```python
from build123d import *

# Parameters (mm, degrees)
EXTRUDE_THIN1_DEPTH = 100
CUT_EXTRUDE2_DEPTH  = 33.5
FILLET1_R           = 3
SKETCH6_W           = 108.670856817
SKETCH6_H           = 17.879774232
CUT_EXTRUDE3_DEPTH  = 166
BOSS_EXTRUDE1_DEPTH = 10.5
CUT_EXTRUDE4_DEPTH  = 27
CUT_EXTRUDE7_DEPTH  = 5
FILLET5_R           = 12


with BuildPart() as part:
    # Sketch1 → Extrude-Thin1 (new body)
    with BuildSketch(Plane(origin=(0, 0, 0), x_dir=(0, 0, -1), z_dir=(1, 0, 0))):
        with BuildLine():
            Line((45, -32), (45, -18))
            ThreePointArc((45, -18), (32.040658091, -6.957616726), (16.501342128, 0))
            ThreePointArc((16.501342128, 0), (0, 1.972757604), (-16.501342128, 0))
            ThreePointArc((-16.501342128, 0), (-32.040658091, -6.957616726), (-45, -18))
            Line((-45, -18), (-45, -32))
            Line((-45, -32), (-48, -32))
            Line((-48, -32), (-48, -16.88185814))
            ThreePointArc((-48, -16.88185814), (-34.099982932, -4.712774746), (-17.26768466, 2.901081048))
            ThreePointArc((-17.26768466, 2.901081048), (0, 4.972757604), (17.26768466, 2.901081048))
            ThreePointArc((17.26768466, 2.901081048), (34.099982932, -4.712774746), (48, -16.88185814))
            Line((48, -16.88185814), (48, -32))
            Line((48, -32), (45, -32))
        make_face()
    extrude(amount=EXTRUDE_THIN1_DEPTH)

    # Sketch5 → Cut-Extrude2 (cut, symmetric)
    with BuildSketch(Plane(origin=(0, 0, 0), x_dir=(1, 0, 0), z_dir=(0, 1, 0))):
        with BuildLine():
            Line((74.78082212, 3), (74.78082212, -3))
            add(Edge.make_bspline(
                [(74.78082212, -3), (97.634090292, -10.562952057), (100, -44)],
                knots=[0, 0, 0, 1, 1, 1], degree=2))
            Line((100, -44), (100, 44))
            add(Edge.make_bspline(
                [(74.78082212, 3), (97.634090292, 10.562952057), (100, 44)],
                knots=[0, 0, 0, 1, 1, 1], degree=2))
        make_face()
    extrude(amount=CUT_EXTRUDE2_DEPTH, both=True, mode=Mode.SUBTRACT)

    # Fillet1
    fillet1_edges = [part.edges().sort_by_distance(p)[0] for p in [
        (50, -16.88185814, -48),
        (50, -16.88185814, 48),
        (74.78082212, 3.409765032, 3),
        (74.78082212, 3.409765032, -3),
        (46.328171757, 2.901081048, -17.26768466),
        (46.328171757, 2.901081048, 17.26768466),
    ]]
    fillet(fillet1_edges, radius=FILLET1_R)

    # Sketch6 → Cut-Extrude3 (cut)
    with BuildSketch(Plane(origin=(0, 0, -48), x_dir=(-1, 0, 0), z_dir=(0, 0, -1))):
        with Locations((-40.664571591, -32.939887116)):
            Rectangle(SKETCH6_W, SKETCH6_H)
    extrude(amount=-CUT_EXTRUDE3_DEPTH, mode=Mode.SUBTRACT)

    # Sketch8 → Boss-Extrude1 (add, symmetric)
    with BuildSketch(Plane.XY):
        Polygon((0, 1.972757604), (-2.848910504, -18), (7.151089496, -18), (15, 1.972757604), align=None)
    extrude(amount=BOSS_EXTRUDE1_DEPTH, both=True)

    # Sketch10 → Cut-Extrude4 (cut)
    with BuildSketch(Plane.XY.offset(10.5)):
        with BuildLine():
            Line((-0.348910504, -18), (3.987157996, -18))
            ThreePointArc((3.987157996, -18), (1.819123746, -14.255159652), (-0.348910504, -18))
        make_face()
    extrude(amount=-CUT_EXTRUDE4_DEPTH, mode=Mode.SUBTRACT)

    # Sketch15 → Cut-Extrude7 (cut)
    with BuildSketch(Plane(origin=(0, 0, -48), x_dir=(-1, 0, 0), z_dir=(0, 0, -1))):
        Polygon((-95, -24), (0, -18.860125055), (0, -26.57204687), align=None)
    cut_extrude7 = extrude(amount=-CUT_EXTRUDE7_DEPTH, mode=Mode.SUBTRACT)

    # Mirror2: Cut-Extrude7 across plane
    add(cut_extrude7.mirror(Plane.XY), mode=Mode.SUBTRACT)

    # Fillet5
    # the kernel refuses this fillet: 12 mm, written as the material it takes off along each edge
    with BuildSketch(Plane(origin=(0, -18.860125055, 76.420758066), x_dir=(0, 1, 0), z_dir=(0, 0, -1))) as fillet5_piece_1:
        with BuildLine():
            CenterArc((FILLET5_R * 0.947358602211, FILLET5_R), FILLET5_R, 183.096908366, 86.903091634)
            Line((-FILLET5_R * 0.0511809847104, FILLET5_R * 0.945975067318), (0, 0))
            Line((0, 0), (FILLET5_R * 0.947358602211, 0))
        make_face()
    extrude(amount=59.841516133, mode=Mode.SUBTRACT)
    with BuildSketch(Plane(origin=(0, -18.860125055, -76.420758066), x_dir=(0, 1, 0), z_dir=(0, 0, 1))) as fillet5_piece_2:
        with BuildLine():
            CenterArc((FILLET5_R * 0.947358602211, -FILLET5_R), FILLET5_R, 90, 86.903091634)
            Line((-FILLET5_R * 0.0511809847104, -FILLET5_R * 0.945975067318), (0, 0))
            Line((0, 0), (FILLET5_R * 0.947358602211, 0))
        make_face()
    extrude(amount=59.841516133, mode=Mode.SUBTRACT)


solid = part.part
```
Geometry: final body of the model. Coordinates: model frame, mm. A direction names the side the tool comes from. Coordinates: 2 decimals unless noted, no trailing zeros. Order: outer loops, then holes, each group sorted by start corner. A loop starts at its lowest first (then second) coordinate and runs counter-clockwise, first axis right, second up. Notation, with made-up numbers: (9, -38.5) -> (39, -38.5) arc R30 cw to (39, -11.5) -> close; hole circle Ø5 at (57.25, 33.5). An arc over 180 degrees is marked (long way). Write each question's results on one line, items separated by ' | '. Start each with the question number.
1) Cut plane B-B, the plane x = 23. Output: boundary loops of the cut face in (y, z).
2) First-contact query: pin 1 (0.9 mm diameter, centred on y = -26.5, z = 47, fed in from -X); pin 2 (2.5 mm diameter, centred on x = 5, z = 5, fed in from -Y); pin 3 (19.5 mm diameter, centred on x = 7, y = -9.5, fed in from +Z); pin 4 (12 mm diameter, centred on x = 34.5, z = 25, fed in from +Y). Flat tips, straight axial feed; report the tip coordinate or a pass-through.
3) Set-up query: faces 1 (the flat face through (67, -21, 45)), 2 (the cylindrical face through (2.39, -14.68, -43.27)), 3 (the cylindrical face through (2.444, -14.75, 43.273)). Return all of +Z, -Z, +X, -X, +Y, -Y with unobstructed straight access to the full face (end or side cutting, diameter ignored); none if empty.
4) Cut plane C-C, the plane y = -3. State how many separate pieces and enclosed holes the cut face has, and give its area (3 significant figures).
5) Mould query, pull axis Z, two halves, no side actions, for faces 4 (the cylindrical face through (49.3, -6.83, 31.84)), 5 (the cylindrical face through (45.68, 4.972, 0.244)), 6 (the flat face through (-2, -18, 0)). Classes: released by +Z, released by -Z, zero draft, split by the parting line, or undercut.
6) Cut plane A-A, the plane y = -28.5. Output: boundary loops of the cut face in (x, z).
7) Material intervals for line 1 along Z through (x, y) = (60, -16.5); line 2 along Y through (x, z) = (38.5, -22.5); line 3 along X through (y, z) = (-1.5, 5), sorted ascending.
8) Cut plane D-D, the plane x = 73. Output: boundary loops of the cut face in (y, z).
Checks:
1) outline: (-20.1, -48) -> (-18, -48) arc R3 ccw to (-16.02, -47.25) arc R63 ccw to (2.9, -17.27) arc R73 ccw to (2.9, 17.27) arc R63 ccw to (-16.02, 47.25) arc R3 ccw to (-18, 48) -> (-20.1, 48) -> (-20.1, 45) -> (-18, 45) arc R60 cw to (0, 16.5) arc R70 cw to (0, -16.5) arc R60 cw to (-18, -45) -> (-20.1, -45) -> close
2) pin 1: x = 95 | pin 2: y = -18 | pin 3: z = 48 | pin 4: y = 2.38
3) face 1: +X, -X, -Y | face 2: -Z, -X, -Y | face 3: +Z, -X, -Y
4) separate pieces: 3 | enclosed holes: 0 | area: 1,570 mm^2
5) face 4: undercut | face 5: split by the parting line | face 6: zero draft
6) outline: (95, -48) -> (100, -48) -> (100, -45) -> (95, -45) -> close; (95, 45) -> (100, 45) -> (100, 48) -> (95, 48) -> close
7) line 1: -47.6 to -43.63, 43.63 to 47.6 | line 2: -2.06 to 1.16 | line 3: -0.5 to 13.64
8) outline: (-22.81, -48) -> (-18, -48) arc R3 ccw to (-16.02, -47.25) arc R63 ccw to (2.9, -17.27) arc R73 ccw to (2.9, 17.27) arc R63 ccw to (-16.02, 47.25) arc R3 ccw to (-18, 48) -> (-22.81, 48) -> (-22.81, 45) -> (-18, 45) arc R60 cw to (0, 16.5) arc R70 cw to (0, -16.5) arc R60 cw to (-18, -45) -> (-22.81, -45) -> close
